Part model, mm, in its own coordinate system. A direction names the side the tool comes from. Coordinates: 2 decimals unless noted, no trailing zeros. Order: outer loops, then holes, each group sorted by start corner. A loop starts at its lowest first (then second) coordinate and runs counter-clockwise, first axis right, second up. Notation, with made-up numbers: (84, 23) - (89, 23) arc R18 ccw to (89, 29) - close; hole circle Ø10 at (48, 47.5). An arc over 180 degrees is marked (long way). Use a Markdown table: item, result. Add a question column.
1) Tool access for faces 4 (the face through (-7.093, -8, 4)), 5 (the face through (1, -8, 8.362)), 6 (the face through (0.15, -5.41, 3.23)): list every direction of +Z, -Z, +X, -X, +Y, -Y with a clear straight run to the whole face (end or side of a thin tool).
2) Wall check: L1, parallel to Y at x = 4.25, z = 3.5; L2, parallel to X at y = -13.25, z = 0.25; L3, parallel to Y at x = 2.5, z = 6.5. Give the ranges that are in metal, low to high. Write a range as [from, to].
3) Saw through at B-B on z = 6.75. List the corners of the cut face in (x, y), then the cut area to 3 significant figures.
4) Saw through at A-A on y = -4.13. List the corners of the cut face in (x, z), then the cut area to 3 significant figures.
5) Two-plate mould, pull along Y, no slides. Class faces 1 (the face through (2.55, -5.615, 9.298)), 2 (the face through (-3, -4, 10.262)), 3 (the face through (1, -15.71, 4)): +Y half, -Y half, draft (parallel to the pull), parting line (faces both ways), or undercut.
6) Saw through at C-C on y = -2.25. List the corners of the cut face in (x, z).
```python
from build123d import *

# Parameters (mm, degrees)
F0_W     = 15.71
F0_H     = 9.57
F1_DEPTH = 15.71
F2_R     = 2.44
F3_DEPTH = 1.9
F4_W     = 13.29
F4_H     = 13.29
F4_R     = 2
F4_R_2   = 3.24
F5_DEPTH = 9
F6_R     = 2.48
F7_DEPTH = 9


with BuildPart() as f1:
    # F0 (on Front) → F1 (new body)
    with BuildSketch(Plane.XZ):
        with Locations((0.7616067305, 3.5766704181)):
            Rectangle(F0_W, F0_H)
    extrude(amount=F1_DEPTH)

    # F2 (on face) → F3 (join)
    with BuildSketch(Plane.XY.offset(8.3616704181)):
        with Locations((4.4866067305, -11.58)):
            Circle(F2_R)
        with Locations((-2.9633932695, -11.58)):
            Circle(F2_R)
        with Locations((-2.9633932695, -4.13)):
            Circle(F2_R)
        with Locations((4.4866067305, -4.13)):
            Circle(F2_R)
    extrude(amount=F3_DEPTH)

    # F4 (on face) → F5 (cut)
    with BuildSketch(Plane(origin=(0, 0, -1.2083295819), x_dir=(1, 0, 0), z_dir=(0, 0, -1))):
        with Locations((0.7616067305, 7.855)):
            Rectangle(F4_W, F4_H)
        with Locations((-3.647951686, 3.4200778348)):
            Circle(F4_R, mode=Mode.SUBTRACT)
        with Locations((0.6830992061, 7.8338431194)):
            Circle(F4_R_2, mode=Mode.SUBTRACT)
        with Locations((5.201886408, 3.4736101516)):
            Circle(F4_R, mode=Mode.SUBTRACT)
        with Locations((-3.6477285673, 12.270077832)):
            Circle(F4_R, mode=Mode.SUBTRACT)
        with Locations((5.2021095268, 12.3236101487)):
            Circle(F4_R, mode=Mode.SUBTRACT)
        with Locations((-3.647951686, 3.4200778348)):
            Circle(F4_R)
        with Locations((-3.6477285673, 12.270077832)):
            Circle(F4_R)
        with Locations((5.2021095268, 12.3236101487)):
            Circle(F4_R)
        with Locations((5.201886408, 3.4736101516)):
            Circle(F4_R)
    extrude(amount=-F5_DEPTH, mode=Mode.SUBTRACT)

    # F6 (on face) → F7 (cut)
    with BuildSketch(Plane(origin=(0, 0, -1.2083295819), x_dir=(1, 0, 0), z_dir=(0, 0, -1))):
        with Locations((0.6830992061, 7.8338431194)):
            Circle(F6_R)
    extrude(amount=-F7_DEPTH, mode=Mode.SUBTRACT)


solid = f1.part
```
Results are:
| question | item | result |
|---|---|---|
| 1 | face 4 | +Z, -Z, -X, +Y, -Y |
| 1 | face 5 | +Z |
| 1 | face 6 | -Z |
| 2 | L1 | [-15.71, -14.5], [-1.21, 0] |
| 2 | L2 | [-7.09, -5.88], [7.41, 8.62] |
| 2 | L3 | [-15.71, -14.5], [-10.52, -9.52], [-6.15, -5.15], [-1.21, 0] |
| 3 | outline | (-7.09, -15.71) - (8.62, -15.71) - (8.62, 0) - (-7.09, 0) - close; circle Ø6.48 at (0.68, -7.83); hole (-5.88, -14.5) - (7.41, -14.5) - (7.41, -1.21) - (-5.88, -1.21) - close; hole circle Ø4.96 at (0.68, -7.83) |
| 3 | area | 83.8 mm2 |
| 4 | outline | (-7.09, -1.21) - (-5.88, -1.21) - (-5.88, 7.79) - (7.41, 7.79) - (7.41, -1.21) - (8.62, -1.21) - (8.62, 8.36) - (6.93, 8.36) - (6.93, 10.26) - (2.05, 10.26) - (2.05, 8.36) - (-0.52, 8.36) - (-0.52, 10.26) - (-5.4, 10.26) - (-5.4, 8.36) - (-7.09, 8.36) - close |
| 4 | area | 49.3 mm2 |
| 5 | face 1 | undercut |
| 5 | face 2 | draft |
| 5 | face 3 | -Y half |
| 6 | outline | (-7.09, -1.21) - (-5.88, -1.21) - (-5.88, 7.79) - (7.41, 7.79) - (7.41, -1.21) - (8.62, -1.21) - (8.62, 8.36) - (6.04, 8.36) - (6.04, 10.26) - (2.93, 10.26) - (2.93, 8.36) - (-1.41, 8.36) - (-1.41, 10.26) - (-4.52, 10.26) - (-4.52, 8.36) - (-7.09, 8.36) - close |
